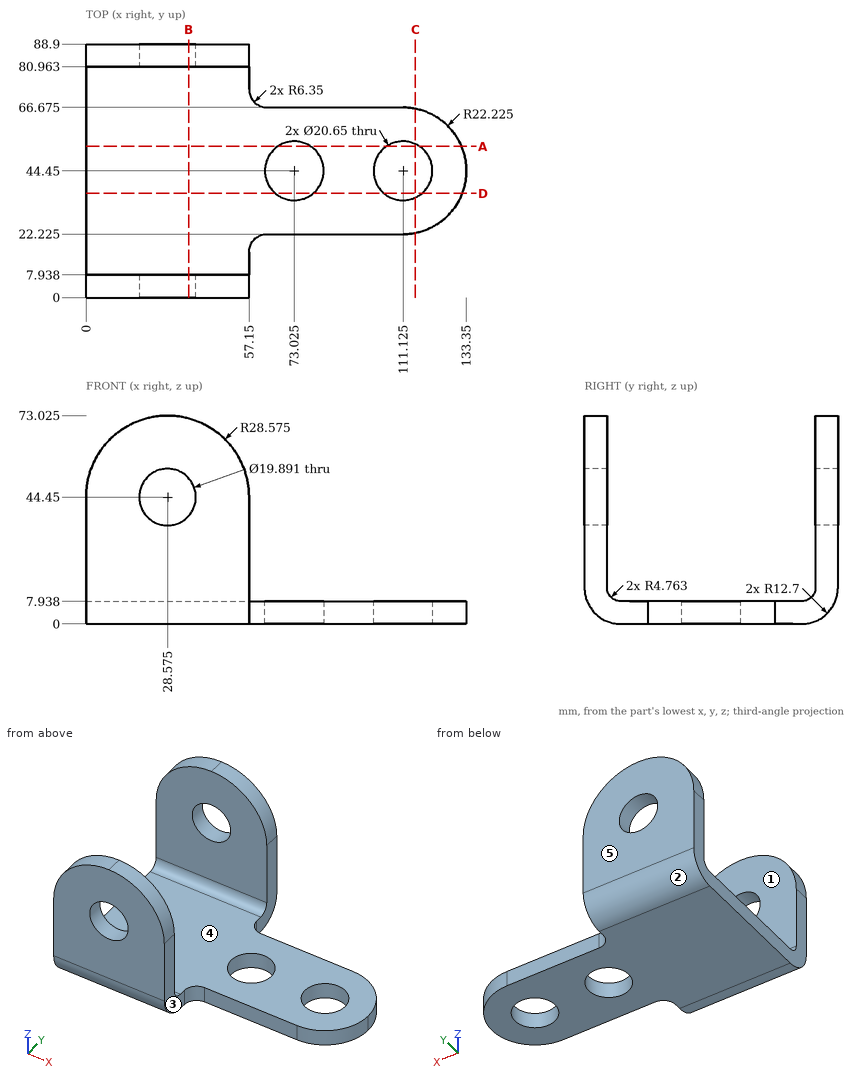
Geometry: see drawing. Coordinates: mm, zero at the bounding-box minimum. A direction names the side the tool comes from. Coordinates: 2 decimals unless noted, no trailing zeros. Loops run counter-clockwise (first coordinate to the right, second up) from the corner with the lowest first, then second, coordinate; pieces in that order, holes last.
Q1. Cut plane C-C (x = 115.5). Output: boundary loops of the cut face in (y, z).
Q2. Cut plane B-B (x = 36). Output: boundary loops of the cut face in (y, z) (1 decimal).
Q3. Cut plane D-D (y = 36.5). Output: boundary loops of the cut face in (x, z).
Q4. Cut plane A-A (y = 53). Output: boundary loops of the cut face in (x, z), then the cut area to 3 significant figures.
Q5. Contact query for flat-ended pins moving along their axis: pin 1 (16 mm diameter, centred on x = 28.575, z = 44.45, fed in from +Y); pin 2 (6 mm diameter, centred on x = 60.5, y = 33.5, fed in from +Z); pin 3 (4 mm diameter, centred on x = 97.5, z = 3, fed in from -Y) (1 decimal); pin 4 (12.5 mm diameter, centred on y = 5, z = 12, fed in from +X). Output: stop coordinate, or through.
Q6. Material intervals for line 1 (X direction, y = 44, z = 6) (1 decimal); line 2 (Y direction, x = 47, z = 40); line 3 (Z direction, x = 27, y = 54.5), sorted ascending.
Q7. Set-up query: the marked faces 4 and 5. Return all of +Z, -Z, +X, -X, +Y, -Y with unobstructed straight access to the full face (end or side cutting, diameter ignored); none if empty.
Q8. Draft query along Y for the marked faces 1, 2 and 3. Return one class per face: +Y half, -Y half, draft (parallel to the pull), parting line (faces both ways), or undercut.
Working result:
1. outline: (22.66, 0) - (35.1, 0) - (35.1, 7.94) - (22.66, 7.94) - close; (53.8, 0) - (66.24, 0) - (66.24, 7.94) - (53.8, 7.94) - close
2. outline: (0, 12.7) arc R12.7 ccw to (12.7, 0) - (76.2, 0) arc R12.7 ccw to (88.9, 12.7) - (88.9, 37.8) - (81, 37.8) - (81, 12.7) arc R4.8 cw to (76.2, 7.9) - (12.7, 7.9) arc R4.8 cw to (7.9, 12.7) - (7.9, 37.8) - (0, 37.8) - close; (0, 51.1) - (7.9, 51.1) - (7.9, 72) - (0, 72) - close; (81, 51.1) - (88.9, 51.1) - (88.9, 72) - (81, 72) - close
3. outline: (0, 0) - (66.44, 0) - (66.44, 7.94) - (0, 7.94) - close; (79.61, 0) - (104.54, 0) - (104.54, 7.94) - (79.61, 7.94) - close; (117.71, 0) - (131.88, 0) - (131.88, 7.94) - (117.71, 7.94) - close
4. outline: (0, 0) - (67.24, 0) - (67.24, 7.94) - (0, 7.94) - close; (78.81, 0) - (105.34, 0) - (105.34, 7.94) - (78.81, 7.94) - close; (116.91, 0) - (131.64, 0) - (131.64, 7.94) - (116.91, 7.94) - close
4. area: 861 mm2
5. pin 1: passes through
5. pin 2: stops at z = 7.94
5. pin 3: stops at y = 22.2
5. pin 4: stops at x = 57.15
6. line 1: x = 0 to 62.7, 83.3 to 100.8, 121.4 to 133.3
6. line 2: y = 0 to 7.94, 80.96 to 88.9
6. line 3: z = 0 to 7.94
7. face 4: +Z, +X, -X
7. face 5: +Z, -Z, +X, -X, +Y
8. face 1: undercut
8. face 2: +Y half
8. face 3: draft
